```python
from build123d import *

# Parameters (mm, degrees)
F0_W     = 635
F0_H     = 1270
F1_DEPTH = 50.8
F2_R     = 75
F3_DEPTH = 347


with BuildPart() as f1:
    # F0 (on Top) → F1 (new body)
    with BuildSketch(Plane.XY):
        with Locations((136.374186, 280.478615)):
            Rectangle(F0_W, F0_H)
    extrude(amount=F1_DEPTH)

    # F2 (on face) → F3 (cut)
    with BuildSketch(Plane(origin=(0, 0, 0), x_dir=(1, 0, 0), z_dir=(0, 0, -1))):
        with Locations((303.242054, 250)):
            Circle(F2_R)
        with Locations((303.242054, 0)):
            Circle(F2_R)
        with Locations((303.242054, -250)):
            Circle(F2_R)
    extrude(amount=-F3_DEPTH, mode=Mode.SUBTRACT)


solid = f1.part
```
CAD build for the part. Positions are in the model's coordinates, mm. Round coordinates to 2 decimals unless told otherwise and drop trailing zeros. Order: outer loops, then holes, each group sorted by start corner. A loop starts at its lowest first (then second) coordinate and runs counter-clockwise, first axis right, second up.
Item 1: Saw through at D-D on y = 37. Write the cut outline in (x, z).
Item 2: Saw through at A-A on y = -250. Write the cut outline in (x, z), then the cut area to 3 significant figures.
Item 3: Mould opens along Y. For faces 1 (the face through (132, 289, 0)), 2 (the face through (374.78, -272.53, 25.04)), 3 (the face through (132, 915.479, 25)) say: pulls with the +Y half, pulls with the -Y half, needs draft (parallel to the pull), parting line crosses it, or undercut.
Item 4: Saw through at C-C on x = 300. Write the cut outline in (y, z), then the cut area to 3 significant figures.
Item 5: Saw through at B-B on z = 43. Write the cut outline in (x, y), then the cut area to 3 significant figures.
Item 6: Probe line 1 along Y through (x, z) = (272.5, 17.5); line 2 along Y through (x, z) = (321.5, 16.5); line 3 along X through (y, z) = (0, 19). List the from-to ranges inside material, lowest first.
Reported:
1. outline: (-181.13, 0) - (238, 0) - (238, 50.8) - (-181.13, 50.8) - close; (368.48, 0) - (453.87, 0) - (453.87, 50.8) - (368.48, 50.8) - close
2. outline: (-181.13, 0) - (228.24, 0) - (228.24, 50.8) - (-181.13, 50.8) - close; (378.24, 0) - (453.87, 0) - (453.87, 50.8) - (378.24, 50.8) - close
2. area: 24,600 mm2
3. face 1: needs draft
3. face 2: undercut
3. face 3: pulls with the +Y half
4. outline: (-354.52, 0) - (-324.93, 0) - (-324.93, 50.8) - (-354.52, 50.8) - close; (-175.07, 0) - (-74.93, 0) - (-74.93, 50.8) - (-175.07, 50.8) - close; (74.93, 0) - (175.07, 0) - (175.07, 50.8) - (74.93, 50.8) - close; (324.93, 0) - (915.48, 0) - (915.48, 50.8) - (324.93, 50.8) - close
4. area: 41,700 mm2
5. outline: (-181.13, -354.52) - (453.87, -354.52) - (453.87, 915.48) - (-181.13, 915.48) - close; hole circle Ø150 at (303.24, -250); hole circle Ø150 at (303.24, 0); hole circle Ø150 at (303.24, 250)
5. area: 753,000 mm2
6. line 1: y = -354.52 to -318.41, -181.59 to -68.41, 68.41 to 181.59, 318.41 to 915.48
6. line 2: y = -354.52 to -322.74, -177.26 to -72.74, 72.74 to 177.26, 322.74 to 915.48
6. line 3: x = -181.13 to 228.24, 378.24 to 453.87
